```python
from build123d import *

# Parameters (mm, degrees)
SKETCH1_R           = 10
SKETCH1_R_2         = 9
BOSS_EXTRUDE1_DEPTH = 160
SKETCH3_R           = 10
SKETCH7_R           = 10


with BuildPart() as part:
    # Sketch1 → Boss-Extrude1 (new body)
    with BuildSketch(Plane.XY):
        Circle(SKETCH1_R)
        Circle(SKETCH1_R_2, mode=Mode.SUBTRACT)
    extrude(amount=-BOSS_EXTRUDE1_DEPTH)

    # Sketch3 → Loft3 section 0
    with BuildSketch(Plane.XY, mode=Mode.PRIVATE) as loft3_s0:
        Circle(SKETCH3_R)
    loft([loft3_s0.sketch, Vertex(0, 0, 30)])

    # Sketch7 → Loft4 section 0
    with BuildSketch(Plane(origin=(0, 0, -160), x_dir=(-1, 0, 0), z_dir=(0, 0, -1)), mode=Mode.PRIVATE) as loft4_s0:
        Circle(SKETCH7_R)
    loft([loft4_s0.sketch, Vertex(0, 0, -190)])


solid = part.part
```
Source: CAD feature listing. Evaluate the final solid. Frame: model axes, mm. A direction names the side the tool comes from. Give positions to 0.01 mm unless a question says otherwise; leave off trailing zeros. Order: outer loops, then holes, each group sorted by start corner. A loop starts at its lowest first (then second) coordinate and runs counter-clockwise, first axis right, second up.
(1) Section query B-B (z = -163.5). Return the cut outline in (x, y).
(2) Access query for faces 1 (the face through (-1.069, -4.813, 15.21)), 2 (the face through (0, 0, -160)). Directions: +Z, -Z, +X, -X, +Y, -Y. A direction counts if a zero-diameter tool reaches every point of the face in a straight line with its end or side. Return the directions, or none.
(3) Pull-direction query (Y, two-part tool) for faces 3 (the face through (1.069, -4.813, -175.21)), 4 (the face through (-1.172, 8.923, -78.88)); classes: +Y half, -Y half, draft (parallel to the pull), parting line (faces both ways), or undercut.
(4) Section query A-A (z = -124). Return the cut outline in (x, y).
(5) Contact query for flat-ended pins moving along their axis: P1, Ø1.5, axis at y = 4, z = -72.5, coming from the -X side; P2, Ø1, axis at x = -5, z = -129.5, coming from the -Y side; P3, Ø8, axis at x = -6.5, z = -93, coming from the -Y side. Output: stop coordinate, or through.
(6) Material intervals for line 1 along Y through (x, z) = (0, -79); line 2 along X through (y, z) = (-3.25, -74); line 3 along Y through (x, z) = (5.5, -71), sorted ascending.
Outcome:
1. outline: circle Ø17.67 at (0, 0)
2. face 1: +Z
2. face 2: none
3. face 3: parting line
3. face 4: undercut
4. outline: circle Ø20 at (0, 0); hole circle Ø18 at (0, 0)
5. P1: stops at x = -9.46
5. P2: stops at y = -8.93
5. P3: stops at y = -9.68
6. line 1: y = -10 to -9, 9 to 10
6. line 2: x = -9.46 to -8.39, 8.39 to 9.46
6. line 3: y = -8.35 to -7.12, 7.12 to 8.35
